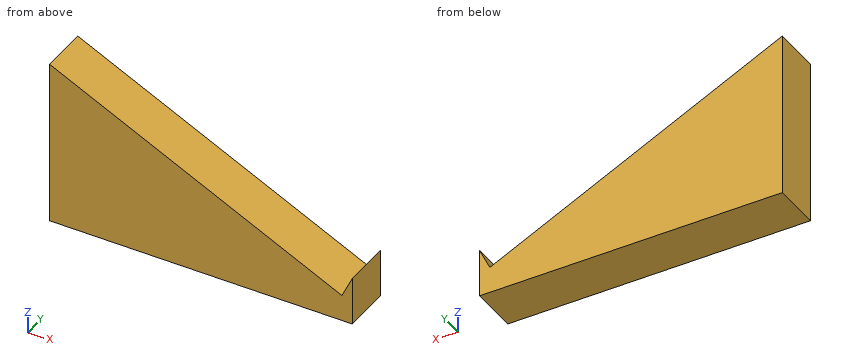
from build123d import *

# Parameters (mm, degrees)
F1_DEPTH = 5
F2_DEPTH = 2.5


with BuildPart() as f1:
    # F0 (on Front) → F1 (new body)
    with BuildSketch(Plane.XZ):
        Polygon((0, 20), (0, 0), (31.3749988316, 0), (31.3749988316, 5), align=None)
    extrude(amount=-F1_DEPTH)

    # F2 (cut): a face of the model
    f2_faces = [f1.faces().sort_by_distance(p)[0] for p in [
        (15.6874994158, 2.5, 12.5),
    ]]
    extrude(f2_faces, amount=-F2_DEPTH, mode=Mode.SUBTRACT)


solid = f1.part
Model file for the job. Use its own axes, mm. Round coordinates to 2 decimals unless told otherwise and drop trailing zeros. Loops run counter-clockwise (first coordinate to the right, second up) from the corner with the lowest first, then second, coordinate; pieces in that order, holes last. Notation, with made-up numbers: (37.5, -40) - (55.5, -40) arc R13 ccw to (55.5, -15) - close; hole circle Ø2 at (-6, 57). An arc over 180 degrees is marked (long way). Write each question's results on one line, items separated by ' | '.
(1) Saw through at A-A, the plane z = 3.25. List the corners of the cut face in (x, y) (3 decimals).
Answer below:
outline: (0, 0) - (29.239, 0) - (29.239, 5) - (0, 5) - close; (30.538, 0) - (31.375, 0) - (31.375, 5) - (30.538, 5) - close
(2) Wall check: L1, parallel to X at y = 0.6, z = 3.5 (3 decimals); L2, parallel to X at y = 1.2, z = 4 (3 decimals); L3, parallel to Z at x = 30, y = 0.35. Give the ranges that are in metal, low to high.
Answer below:
L1: x = 0 to 28.716, 30.658 to 31.375 | L2: x = 0 to 27.671, 30.897 to 31.375 | L3: z = 0 to 2.89
(3) Pin check, flat tips, straight feed: pin 1 (8 mm diameter, centred on x = 17, z = 4, fed in from -Y); pin 2 (1 mm diameter, centred on x = 19.5, y = 1.5, fed in from +Z); pin 3 (2 mm diameter, centred on x = 4, y = 1.5, fed in from +Z). Stop position of each tip, or through.
Answer below:
pin 1: stops at y = 0 | pin 2: stops at z = 8.15 | pin 3: stops at z = 15.79
(4) Saw through at B-B, the plane y = 0.8. List the corners of the cut face in (x, z) (3 decimals), then the cut area to 3 significant figures.
Answer below:
outline: (0, 0) - (31.375, 0) - (31.375, 5) - (30.297, 2.745) - (0, 17.229) - close | area: 307 mm^2
(5) Saw through at C-C, the plane x = 4.5. List the corners of the cut face in (y, z).
Answer below:
outline: (0, 0) - (5, 0) - (5, 15.08) - (0, 15.08) - close
(6) Saw through at D-D, the plane z = 14. List the corners of the cut face in (x, y).
Answer below:
outline: (0, 0) - (6.75, 0) - (6.75, 5) - (0, 5) - close
